Could you check a few things on this model? Use its own coordinates, in mm. A direction names the side the tool comes from. Give positions to 0.01 mm unless a question says otherwise; leave off trailing zeros. Write each loop counter-clockwise with the first axis right and the second up, starting at its lowest first coordinate (ties: lowest second). Pieces come first, ordered by that corner, then holes. Notation, with made-up numbers: (-23.75, 83.25) -> (-14.75, 83.25) arc R19 cw to (-14.75, 103.25) -> close; hole circle Ø6 at (-21, 73). An arc over 180 degrees is marked (long way). One line per question, with ' | ' between items.
from build123d import *

# Parameters (mm, degrees)
F0_R     = 9.38
F0_R_2   = 2.5
F1_DEPTH = 5.115
F4_R     = 6.884933
F4_R_2   = 4.503868
F5_DEPTH = 0.5
F6_R     = 6.884933
F6_R_2   = 4.503868
F7_DEPTH = 0.5


with BuildPart() as f1:
    # F0 (on Front) → F1 (new body, symmetric)
    with BuildSketch(Plane.XZ):
        Circle(F0_R)
        Circle(F0_R_2, mode=Mode.SUBTRACT)
    extrude(amount=F1_DEPTH, both=True)

    # F2 (on Right) → F3 (revolve)
    with BuildSketch(Plane.YZ):
        Polygon((-5.115, 9.38), (0, 9.38), (-2.5575, 11.9375), align=None)
        Polygon((2.5575, 11.9375), (0, 9.38), (5.115, 9.38), align=None)
    revolve(axis=Axis((0, 0, 0), (0, 1, 0)))

    # F4 (on face) → F5 (cut)
    with BuildSketch(Plane(origin=(0, 5.115, 0), x_dir=(-1, 0, 0), z_dir=(0, 1, 0))):
        Circle(F4_R)
        Circle(F4_R_2, mode=Mode.SUBTRACT)
    extrude(amount=-F5_DEPTH, mode=Mode.SUBTRACT)

    # F6 (on face) → F7 (cut)
    with BuildSketch(Plane.XZ.offset(5.115)):
        Circle(F6_R)
        Circle(F6_R_2, mode=Mode.SUBTRACT)
    extrude(amount=-F7_DEPTH, mode=Mode.SUBTRACT)


solid = f1.part
Q1. If I drill on line 1 along Z through (x, y) = (0, 4.8) (3 decimals); line 2 along Y through (x, z) = (7.5, 8); line 3 along Z through (x, y) = (0, 4.9) (3 decimals), over which ranges is the centre line in solid material (lowest first)?
Answer below:
line 1: z = -9.695 to -6.885, -4.504 to -2.5, 2.5 to 4.504, 6.885 to 9.695 | line 2: y = -3.53 to -1.59, 1.59 to 3.53 | line 3: z = -9.595 to -6.885, -4.504 to -2.5, 2.5 to 4.504, 6.885 to 9.595
Q2. Imagine slicing it at D-D on y = 1.75. Please give me the cut outline in (x, z).
Answer below:
outline: circle Ø22.26 at (0, 0); hole circle Ø5 at (0, 0)
Q3. Imagine slicing it at C-C on y = -1.25. Please give me the cut outline in (x, z).
Answer below:
outline: circle Ø21.26 at (0, 0); hole circle Ø5 at (0, 0)
Q4. On a 3-axis mill with a long thin cutter (end or side, diameter ignored), from which of +Z, -Z, +X, -X, +Y, -Y can I reach the whole of each face in a straight line? I mean faces 5 (the flat face through (2, 5.115, -2)), 6 (the flat face through (-5, -5.115, 5)), 7 (the conical face through (2.855, 0.124, 9.065)), 8 (the flat face through (-1.4, 4.615, -4.5)), 9 (the flat face through (1.4, -4.615, -4.5)). Say none if no direction works.
Answer below:
face 5: +Z, -Z, +X, -X, +Y | face 6: +Z, -Z, +X, -X, -Y | face 7: none | face 8: +Y | face 9: -Y
Q5. Will these pins go through, and if not, where does the flat tip stop? pin 1 (3 mm diameter, centred on y = 1, z = 0.5, fed in from -X); pin 2 (3 mm diameter, centred on x = 1.5, y = 3, fed in from +Z); pin 3 (3 mm diameter, centred on y = 1, z = 7, fed in from -X).
Answer below:
pin 1: stops at x = -11.87 | pin 2: stops at z = 11.94 | pin 3: stops at x = -9.87
Q6. If we mould it in two halves opening along X, with no side actions, what happens to faces 1 (the flat face through (-5, 5.115, 5)), 2 (the conical face through (-9.31, -0.16, -2.07)), 3 (the cylindrical face through (4.296, -4.868, 1.353)), 4 (the cylindrical face through (-4.296, 4.868, 1.353))? For each: +X half, -X half, draft (parallel to the pull), parting line (faces both ways), or undercut.
Answer below:
face 1: draft | face 2: parting line | face 3: undercut | face 4: undercut
